Geometry: final body of the model. Coordinates: model frame, mm. A direction names the side the tool comes from. Give positions to 0.01 mm unless a question says otherwise; leave off trailing zeros. Write each loop counter-clockwise with the first axis right and the second up, starting at its lowest first coordinate (ties: lowest second). Pieces come first, ordered by that corner, then holes. Notation, with made-up numbers: (50, 74) -> (63, 74) arc R8 cw to (63, 80) -> close; hole circle Ø2 at (11.5, 36). An arc over 180 degrees is marked (long way). Answer as a JSON object with one key per item and string values.
from build123d import *

# Parameters (mm, degrees)
SKETCH1_W           = 50.8
SKETCH1_H           = 38.1
BOSS_EXTRUDE1_DEPTH = 25.4
SKETCH2_W           = 38.1
SKETCH2_H           = 25.4
CUT_EXTRUDE1_DEPTH  = 20.32
SKETCH4_W           = 33.03524
SKETCH4_H           = 3.81762
CUT_EXTRUDE2_DEPTH  = 48.27524
SKETCH5_R           = 1.90881
CUT_EXTRUDE3_DEPTH  = 10.16
CHAMFER1_SIZE       = 0.254
CHAMFER2_SIZE       = 0.254
CUT_EXTRUDE4_REACH  = 39.696
SKETCH15_R          = 1.27


with BuildPart() as part:
    # Sketch1 → Boss-Extrude1 (new body)
    with BuildSketch(Plane(origin=(0, 0, 0), x_dir=(1, 0, 0), z_dir=(0, 1, 0))):
        Rectangle(SKETCH1_W, SKETCH1_H)
    extrude(amount=BOSS_EXTRUDE1_DEPTH)

    # Sketch2 → Cut-Extrude1 (cut)
    with BuildSketch(Plane(origin=(0, 25.4, 0), x_dir=(1, 0, 0), z_dir=(0, 1, 0))):
        Rectangle(SKETCH2_W, SKETCH2_H)
    extrude(amount=-CUT_EXTRUDE1_DEPTH, mode=Mode.SUBTRACT)

    # Sketch4 → Cut-Extrude2 (cut)
    with BuildSketch(Plane.ZY.offset(25.4)):
        with Locations((0, 20.95119)):
            Rectangle(SKETCH4_W, SKETCH4_H)
    extrude(amount=-CUT_EXTRUDE2_DEPTH, mode=Mode.SUBTRACT)

    # Sketch5 → Cut-Extrude3 (cut)
    with BuildSketch(Plane(origin=(0, 25.4, 0), x_dir=(1, 0, 0), z_dir=(0, 1, 0))):
        with Locations(Location((-22.225, 0, 0), (0, 0, 270))):
            Circle(SKETCH5_R)
    extrude(amount=-CUT_EXTRUDE3_DEPTH, mode=Mode.SUBTRACT)

    # Chamfer1
    chamfer1_edges = [part.edges().sort_by_distance(p)[0] for p in [
        (-22.225, 25.4, -1.90881),
    ]]
    chamfer(chamfer1_edges, length=CHAMFER1_SIZE)

    # Chamfer2
    chamfer2_edges = [part.edges().sort_by_distance(p)[0] for p in [
        (-22.225, 19.04238, -1.90881),
    ]]
    chamfer(chamfer2_edges, length=CHAMFER2_SIZE)

    # Sketch15 → Cut-Extrude4 (cut, up to next)
    with BuildSketch(Plane(origin=(0, 5.08, 0), x_dir=(1, 0, 0), z_dir=(0, 1, 0)), mode=Mode.PRIVATE) as cut_extrude4_sk1:
        with Locations(Location((-19.05, 12.7, 0), (0, 0, 270))):
            Circle(SKETCH15_R)
    cut_extrude4_tool1 = extrude(cut_extrude4_sk1.sketch, amount=-CUT_EXTRUDE4_REACH, mode=Mode.PRIVATE) & part.part
    # Sketch15 → Cut-Extrude4 (cut, up to next)
    with BuildSketch(Plane(origin=(0, 5.08, 0), x_dir=(1, 0, 0), z_dir=(0, 1, 0)), mode=Mode.PRIVATE) as cut_extrude4_sk2:
        with Locations(Location((19.05, 12.7, 0), (0, 0, 270))):
            Circle(SKETCH15_R)
    cut_extrude4_tool2 = extrude(cut_extrude4_sk2.sketch, amount=-CUT_EXTRUDE4_REACH, mode=Mode.PRIVATE) & part.part
    # Sketch15 → Cut-Extrude4 (cut, up to next)
    with BuildSketch(Plane(origin=(0, 5.08, 0), x_dir=(1, 0, 0), z_dir=(0, 1, 0)), mode=Mode.PRIVATE) as cut_extrude4_sk3:
        with Locations(Location((-19.05, -12.7, 0), (0, 0, 90))):
            Circle(SKETCH15_R)
    cut_extrude4_tool3 = extrude(cut_extrude4_sk3.sketch, amount=-CUT_EXTRUDE4_REACH, mode=Mode.PRIVATE) & part.part
    # Sketch15 → Cut-Extrude4 (cut, up to next)
    with BuildSketch(Plane(origin=(0, 5.08, 0), x_dir=(1, 0, 0), z_dir=(0, 1, 0)), mode=Mode.PRIVATE) as cut_extrude4_sk4:
        with Locations(Location((19.05, -12.7, 0), (0, 0, 90))):
            Circle(SKETCH15_R)
    cut_extrude4_tool4 = extrude(cut_extrude4_sk4.sketch, amount=-CUT_EXTRUDE4_REACH, mode=Mode.PRIVATE) & part.part
    add(cut_extrude4_tool1.solids().sort_by_distance((-19.05, 5.08, -12.7))[0], mode=Mode.SUBTRACT)
    add(cut_extrude4_tool2.solids().sort_by_distance((19.05, 5.08, -12.7))[0], mode=Mode.SUBTRACT)
    add(cut_extrude4_tool3.solids().sort_by_distance((-19.05, 5.08, 12.7))[0], mode=Mode.SUBTRACT)
    add(cut_extrude4_tool4.solids().sort_by_distance((19.05, 5.08, 12.7))[0], mode=Mode.SUBTRACT)


solid = part.part
Q1. Cut plane B-B (z = 0). Return the cut outline in (x, y).
Values:
{"outline": "(-25.4, 0) -> (25.4, 0) -> (25.4, 25.4) -> (19.05, 25.4) -> (19.05, 22.86) -> (22.88, 22.86) -> (22.88, 19.04) -> (19.05, 19.04) -> (19.05, 5.08) -> (-19.05, 5.08) -> (-19.05, 19.04) -> (-20.06, 19.04) -> (-20.32, 18.79) -> (-20.32, 15.24) -> (-24.13, 15.24) -> (-24.13, 18.79) -> (-24.39, 19.04) -> (-25.4, 19.04) -> close; (-25.4, 22.86) -> (-24.13, 22.86) -> (-24.13, 25.15) -> (-24.39, 25.4) -> (-25.4, 25.4) -> close; (-20.32, 22.86) -> (-19.05, 22.86) -> (-19.05, 25.4) -> (-20.06, 25.4) -> (-20.32, 25.15) -> close"}
Q2. Cut plane D-D (x = -3). Return the cut outline in (y, z), and give its area (3 significant figures).
Values:
{"outline": "(0, -19.05) -> (25.4, -19.05) -> (25.4, -12.7) -> (22.86, -12.7) -> (22.86, -16.52) -> (19.04, -16.52) -> (19.04, -12.7) -> (5.08, -12.7) -> (5.08, 12.7) -> (19.04, 12.7) -> (19.04, 16.52) -> (22.86, 16.52) -> (22.86, 12.7) -> (25.4, 12.7) -> (25.4, 19.05) -> (0, 19.05) -> close", "area": "422 mm²"}
Q3. First-contact query: P1, Ø1.5, axis at x = -19.05, z = -12.7, coming from the -Y side; P2, Ø3, axis at x = -22.225, z = 0, coming from the -Y side; P3, Ø10, axis at x = -5, z = 6.5, coming from the +Y side. Flat tips, straight axial feed; report the tip coordinate or a pass-through.
Values:
{"P1": "y = 5.08", "P2": "y = 0", "P3": "y = 5.08"}
Q4. Cut plane A-A (z = -10). Return the cut outline in (x, y), and give its area (3 significant figures).
Values:
{"outline": "(-25.4, 0) -> (25.4, 0) -> (25.4, 25.4) -> (19.05, 25.4) -> (19.05, 22.86) -> (22.88, 22.86) -> (22.88, 19.04) -> (19.05, 19.04) -> (19.05, 5.08) -> (-19.05, 5.08) -> (-19.05, 19.04) -> (-25.4, 19.04) -> close; (-25.4, 22.86) -> (-19.05, 22.86) -> (-19.05, 25.4) -> (-25.4, 25.4) -> close", "area": "477 mm²"}
Q5. Cut plane C-C (y = 8). Return the cut outline in (x, z).
Values:
{"outline": "(-25.4, -19.05) -> (25.4, -19.05) -> (25.4, 19.05) -> (-25.4, 19.05) -> close; hole (-19.05, -12.7) -> (19.05, -12.7) -> (19.05, 12.7) -> (-19.05, 12.7) -> close"}
Q6. Material intervals for L1, parallel to X at y = 16.85, z = 0; L2, parallel to Z at x = -19.05, y = 1.35; L3, parallel to X at y = 2.25, z = 12.7, sorted ascending. Write a range as from..to.
Values:
{"L1": "-25.4..-24.13, -20.32..-19.05, 19.05..25.4", "L2": "-19.05..-13.97, -11.43..11.43, 13.97..19.05", "L3": "-25.4..-20.32, -17.78..17.78, 20.32..25.4"}
Q7. Set-up query: faces 1 (the cylindrical face through (-19.908, 2.576, 13.636)), 2 (the flat face through (-2, 22.86, -15)), 3 (the flat face through (-19.05, 12, 0)), 4 (the flat face through (0, 0, 0)). Return all of +Z, -Z, +X, -X, +Y, -Y with unobstructed straight access to the full face (end or side cutting, diameter ignored); none if empty.
Values:
{"face 1": "-Y", "face 2": "-X", "face 3": "+Y", "face 4": "+Z, -Z, +X, -X, -Y"}
Q8. Mould query, pull axis X, two halves, no side actions, for faces 5 (the flat face through (25.4, 13, 0)), 6 (the flat face through (0, 5.08, 0)), 7 (the flat face through (0, 25.4, -13)). Classes: pulls with the +X half, pulls with the -X half, needs draft (parallel to the pull), parting line crosses it, or undercut.
Values:
{"face 5": "pulls with the +X half", "face 6": "undercut", "face 7": "needs draft"}
